Autodesk Inventor part; units mm, degrees
ref_plane "Work Plane1" through (104.775, 0, 0) normal (0, 0, -1) x (1, 0, 0)
ref_plane "YZ Plane" through (0, 0, 0) normal (1, 0, 0) x (0, 1, 0)
ref_plane "XZ Plane" through (0, 0, 0) normal (0, 1, 0) x (-1, 0, 0)
sketch "Sketch1" plane through (0, 0, 0) normal (0, 0, 1) x (1, 0, 0)
  line L0 (16, 0) -> (16, 2)
  line L1 (16, 2) -> (5, 2)
  line L2 (5, 2) -> (4.5706, 2)
  line L3 (0, 3.765) -> (0, 1.4434)
  line L4 (0, 1.4434) -> (1.78, 1.4434)
  line L5 (1.78, 1.4434) -> (2.6133, 0)
  line L6 (2.6133, 0) -> (16, 0)
  line L7 (0, 3.765) -> (0.715, 3.765)
  line L8 (0.715, 3.765) -> (2.48, 2)
  line L9 (4.5706, 2) -> (2.48, 2)
  line L10 (5, 2) -> (2.48, 2) construction
  line L11 (2.48, 2) -> (2.48, 2)
  line L12 (-3.2, 0) -> (19.2, 0)
  line L13 (0, -0.753) -> (0, 4.518)
  dimension "d0" = 16
  dimension "d1" = 11
  dimension "d2" = 1.78
  dimension "d3" = 4
  dimension "d6" = 2.48
  dimension "d7" = 45
  dimension "d8" = 2.8868
  dimension "d9" = 60
  dimension "d10" = 7.53
  dimension "d11" = 4
  dimension "d12" = 0.4294
revolve "Body" add sketch "Sketch1" angle 360 about axis through (2.6133, 0, 0) along (1, 0, 0) contours L6 L5 L4 L3 L7 L8 L9 L2 L1 L0
sketch "Sketch2" plane through (0, 0, 0) normal (-1, 0, 0) x (0, 0, 1)
  circle A0 centre (0, 0) radius 1.4434
  line L0 (0, -5.271) -> (0, 5.271)
  line L1 (-5.271, 0) -> (5.271, 0)
  line L2 (1.4434, 0) -> (0.7217, -1.25)
  line L3 (0.7217, -1.25) -> (-0.7217, -1.25)
  line L4 (-0.7217, -1.25) -> (-1.4434, 0)
  line L5 (-1.4434, 0) -> (-0.7217, 1.25)
  line L6 (-0.7217, 1.25) -> (0.7217, 1.25)
  line L7 (0.7217, 1.25) -> (1.4434, 0)
  point P0 (0, 1.4434)
extrude "Slot" add sketch "Sketch2" against normal up to next contours L7 A0 | A0 L2 | L6 L0 A0 | A0 L0 L3 | L0 L6 A0 | A0 L3 L0 | L4 A0 | A0 L5
thread "Thread"
chamfer "Chamfer1" distance 0.4294 distance2 0.4294 1 edges at (16, -2, 0) measured on face at (16, 0.2227, -0.5871)
ref_plane "Work Plane1" through (104.775, 0, 0) normal (0, 0, -1) x (1, 0, 0)
equation "\"d15\" = GEL"
equation "\"d17\" = -0.5 * SPD + 0.5 * GD"
equation "\"d18\" = GUL"
equation "\"d0\" = NLG"
equation "\"d1\" = GEL"
equation "\"d2\" = INTI"
equation "\"d3\" = GD"
equation "\"d6\" = KOH"
equation "\"d7\" = 0.5 * SEWI"
equation "\"d8\" = 1.1547 * SW"
equation "\"d10\" = KOD"
equation "\"d11\" = BDM"
equation "\"d12\" = GAL"
equation "\"NLG\" = 16"
equation "\"INTI\" = 1.78"
equation "\"GEL\" = 11"
equation "\"GAL\" = 0.61345 * PTC"
equation "\"KOH\" = 2.48"
equation "\"KOD\" = 7.53"
equation "\"GUL\" = 0.61345 * PTC"
equation "\"SPD\" = NND - 1.2269 * PTC"
equation "\"BDM\" = NND"
equation "\"GD\" = NND"
equation "\"SEWI\" = 90deg"
equation "\"SW\" = 2.5"
equation "\"TOA\" = 30deg"
equation "\"GD1\" = THREADDIA - 1.2269 * PTC"
equation "\"EPV\" = 4.48"
equation "\"THREADDIA\" = 4"
equation "\"PTC\" = 0.7"
equation "\"NND\" = 4"
equation "\"E0\" = 2.89"
equation "\"THREADDESC\" = 1.2345"
properties part number "ISO 10642 - M4 x  16" material "Steel"
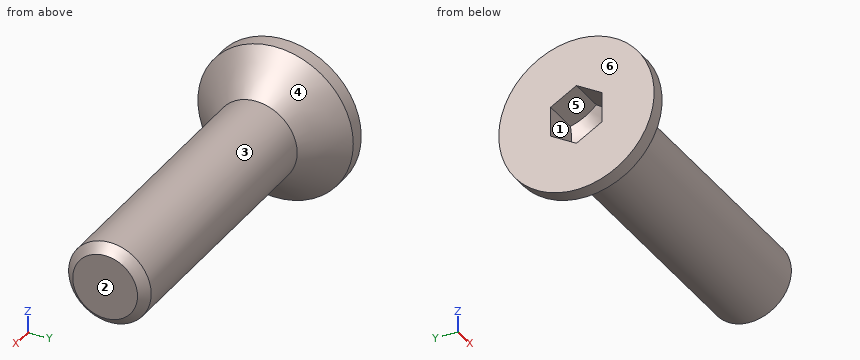
For this review, take the finished solid that the model builds, in its own axes (mm). Face numbers are marked on the shaded views. A direction names the side the tool comes from. Round coordinates to 2 decimals unless told otherwise and drop trailing zeros. Loops run counter-clockwise (first coordinate to the right, second up) from the corner with the lowest first, then second, coordinate; pieces in that order, holes last. Notation, with made-up numbers: (-22.75, 12.5) - (-1.75, 12.5) arc R25 ccw to (-1.75, 50.5) - close; hole circle Ø8 at (68.25, 20.5). An arc over 180 degrees is marked (long way). Put each result on its own line as item: value. Start each with the question number.
1. Consider section A-A on x = 11.75. State the section outline as (y, z) points, plus the area to 3 significant figures.
2. Insertion check: P1, Ø3, axis at y = -2, z = 2.5, coming from the +X side; P2, Ø1.5, axis at x = 12, y = -1, coming from the +Z side; P3, Ø1, axis at y = -2.5, z = 2.5, coming from the +X side. Each pin has a flat end and moves straight along its axis. Give the tip position at first contact, or say it passes through.
3. For probe 1 along X at (y, z) = (0.5, 0.75); probe 2 along X at (y, z) = (0.5, -3); probe 3 along Z at (x, y) = (3.5, 0.5), list the stretches that pass through material, from the lowest coordinate up. Write a range as [from, to].
4. Mouldability with a two-part tool opening along Y and no side actions: class the marked faces 4, 5 and 6 as +Y half, -Y half, draft (parallel to the pull), parting line (faces both ways), or undercut.
5. For the marked faces 1, 2 and 3, list the 3-axis set-ups (+Z, -Z, +X, -X, +Y, -Y) from which the entire face can be reached by the end or side of a thin tool; tool diameter is ignored.
Result sheet:
1. outline: circle Ø4 at (0, 0)
1. area: 12.6 mm^2
2. P1: x = 15.87
2. P2: z = 1.98
2. P3: x = 1.44
3. probe 1: [2.09, 16]
3. probe 2: [0, 1.44]
3. probe 3: [-1.94, 1.94]
4. face 4: parting line
4. face 5: undercut
4. face 6: draft
5. face 1: -X
5. face 2: +Z, -Z, +X, +Y, -Y
5. face 3: +X
